Read the model definition and answer for the solid it produces. Units are mm, in the model's axes. A direction names the side the tool comes from. Coordinates: 2 decimals unless noted, no trailing zeros. Loops run counter-clockwise (first coordinate to the right, second up) from the corner with the lowest first, then second, coordinate; pieces in that order, holes last. Notation, with made-up numbers: (48, 69.5) -> (101, 69.5) arc R26 ccw to (101, 93.5) -> close; hole circle Ø2 at (32, 55). An arc over 180 degrees is marked (long way). Answer in a Markdown table with one row per item.
```python
from build123d import *

# Parameters (mm, degrees)
SKETCH_1_R      = 2.1
SKETCH_1_R_2    = 1.1
EXTRUDE_1_DEPTH = 2


with BuildPart() as part:
    # 草图1 → 凸台-拉伸1 (new body)
    with BuildSketch(Plane.XY):
        with BuildLine():
            Line((-65, 27.5), (65, 27.5))
            ThreePointArc((65, 27.5), (72.071067812, 24.571067812), (75, 17.5))
            Line((75, 17.5), (75, -17.5))
            ThreePointArc((75, -17.5), (72.071067812, -24.571067812), (65, -27.5))
            Line((65, -27.5), (-65, -27.5))
            ThreePointArc((-65, -27.5), (-72.071067812, -24.571067812), (-75, -17.5))
            Line((-75, -17.5), (-75, 17.5))
            ThreePointArc((-75, 17.5), (-72.071067812, 24.571067812), (-65, 27.5))
        make_face()
        with Locations((-10, -17.5)):
            Circle(SKETCH_1_R, mode=Mode.SUBTRACT)
        with Locations((10, -17.5)):
            Circle(SKETCH_1_R, mode=Mode.SUBTRACT)
        with Locations((-22.5, 21.5)):
            Circle(SKETCH_1_R_2, mode=Mode.SUBTRACT)
        with Locations((-22.5, 4.5)):
            Circle(SKETCH_1_R_2, mode=Mode.SUBTRACT)
        with Locations((22.5, 4.5)):
            Circle(SKETCH_1_R_2, mode=Mode.SUBTRACT)
        with Locations((22.5, 21.5)):
            Circle(SKETCH_1_R_2, mode=Mode.SUBTRACT)
        with BuildLine():
            Line((-14, 21.5), (14, 21.5))
            ThreePointArc((14, 21.5), (22.5, 13), (14, 4.5))
            Line((14, 4.5), (-14, 4.5))
            ThreePointArc((-14, 4.5), (-22.5, 13), (-14, 21.5))
        make_face(mode=Mode.SUBTRACT)
    extrude(amount=EXTRUDE_1_DEPTH)


solid = part.part
```
1. A tool of negligible diameter and unlimited length cuts with its end or side. For faces 5 (the cylindrical face through (-22.498, 12.813, 0.986)), 6 (the cylindrical face through (71.99, 24.65, 0.99)), from which of +Z, -Z, +X, -X, +Y, -Y can it reach the whole face along a straight path? Write none if from no direction.
A:
| item | result |
|---|---|
| face 5 | +Z, -Z |
| face 6 | +Z, -Z, +X, +Y |
2. Given pin 1 Ø5 at (x, y) = (10, -17.5) entering from +Z; pin 2 Ø1.3 at (x, y) = (-22.5, 4.5) entering from -Z, each flat-ended and moving along its own axis, determine where each tip first touches the part or whether it passes through.
A:
| item | result |
|---|---|
| pin 1 | stops at z = 2 |
| pin 2 | passes through |
3. A cutting plane is placed at B-B on z = 1. Give the vertices of the cut face in (x, y).
A:
| item | result |
|---|---|
| outline | (-75, -17.5) arc R10 ccw to (-65, -27.5) -> (65, -27.5) arc R10 ccw to (75, -17.5) -> (75, 17.5) arc R10 ccw to (65, 27.5) -> (-65, 27.5) arc R10 ccw to (-75, 17.5) -> close; hole circle Ø2.2 at (-22.5, 4.5); hole circle Ø2.2 at (-22.5, 21.5); hole (-14, 4.5) -> (14, 4.5) arc R8.5 ccw to (14, 21.5) -> (-14, 21.5) arc R8.5 ccw to start; hole circle Ø4.2 at (-10, -17.5); hole circle Ø4.2 at (10, -17.5); hole circle Ø2.2 at (22.5, 4.5); hole circle Ø2.2 at (22.5, 21.5) |
4. A cutting plane is placed at A-A on x = 10. Give the vertices of the cut face in (y, z).
A:
| item | result |
|---|---|
| outline | (-27.5, 0) -> (-19.6, 0) -> (-19.6, 2) -> (-27.5, 2) -> close; (-15.4, 0) -> (4.5, 0) -> (4.5, 2) -> (-15.4, 2) -> close; (21.5, 0) -> (27.5, 0) -> (27.5, 2) -> (21.5, 2) -> close |
5. The mould has two halves that part along X. Classify faces 1 (the flat face through (1, 0, 0)), 2 (the cylindrical face through (8.452, -16.081, 0.986)), 3 (the cylindrical face through (72.15, -24.49, 0.99)), 4 (the cylindrical face through (-11.548, -16.081, 0.986)): pulls with the +X half, pulls with the -X half, needs draft (parallel to the pull), parting line crosses it, or undercut.
A:
| item | result |
|---|---|
| face 1 | needs draft |
| face 2 | undercut |
| face 3 | pulls with the +X half |
| face 4 | undercut |
6. Find the intervals of material crossed by probe 1 along Y at (x, z) = (-12.5, 1.85); probe 2 along Y at (x, z) = (-11, 1.05); probe 3 along X at (y, z) = (20.5, 1.55), in increasing order.
A:
| item | result |
|---|---|
| probe 1 | y = -27.5 to 4.5, 21.5 to 27.5 |
| probe 2 | y = -27.5 to -19.35, -15.65 to 4.5, 21.5 to 27.5 |
| probe 3 | x = -74.54 to -22.96, -22.04 to -18, 18 to 22.04, 22.96 to 74.54 |
7. A cutting plane is placed at C-C on y = 8. Give the vertices of the cut face in (x, z).
A:
| item | result |
|---|---|
| outline | (-75, 0) -> (-20.87, 0) -> (-20.87, 2) -> (-75, 2) -> close; (20.87, 0) -> (75, 0) -> (75, 2) -> (20.87, 2) -> close |
